from build123d import *

# Parameters (mm, degrees)
SKETCH2_R           = 42.538
SKETCH2_R_2         = 40.538
BOSS_EXTRUDE1_DEPTH = 51
CUT_EXTRUDE1_DEPTH  = 48
CUT_EXTRUDE3_START  = -1
CUT_EXTRUDE3_DEPTH  = 1
SKETCH29_R          = 10.65
CUT_EXTRUDE16_DEPTH = 1
CUT_EXTRUDE17_START = -2
SKETCH30_R          = 42.538
SKETCH30_R_2        = 41.538
CUT_EXTRUDE17_DEPTH = 2
BOSS_EXTRUDE3_DEPTH = 1
BOSS_EXTRUDE4_START = 1
SKETCH33_R          = 42.538
SKETCH33_R_2        = 41.638
BOSS_EXTRUDE4_DEPTH = 1


# Read off the part's stored shape, not the designer's step: Cut-Extrude3
with BuildPart() as part:
    # Sketch2 → Boss-Extrude1 (new body)
    with BuildSketch(Plane(origin=(0, 0, 0), x_dir=(-1, 0, 0), z_dir=(0, 1, 0))):
        with Locations(Location((-29.391570254, 2.611368154, 0), (0, 0, 90))):
            Circle(SKETCH2_R)
        with Locations(Location((-29.391570254, 2.611368154, 0), (0, 0, 90))):
            Circle(SKETCH2_R_2, mode=Mode.SUBTRACT)
    extrude(amount=BOSS_EXTRUDE1_DEPTH)

    # Sketch3 → Cut-Extrude1 (cut)
    with BuildSketch(Plane.XY):
        with BuildLine():
            Line((17.725570254, 19.5), (17.725570254, 51))
            Line((17.725570254, 51), (41.057570254, 51))
            Line((41.057570254, 51), (41.057570254, 19.5))
            ThreePointArc((41.057570254, 19.5), (29.391570254, 7.834), (17.725570254, 19.5))
        make_face()
    extrude(amount=CUT_EXTRUDE1_DEPTH, mode=Mode.SUBTRACT)

    # Cut-Extrude3 outline → Cut-Extrude3 (cut)
    with BuildSketch(Plane(origin=(0, 51, 0), x_dir=(1, 0, 0), z_dir=(0, 1, 0)).offset(CUT_EXTRUDE3_START)):
        with BuildLine():
            ThreePointArc((41.057570254, -43.518407744), (29.391570254, 39.926631846), (17.725570254, -43.518407744))
            Line((17.725570254, -43.518407744), (17.725570254, -41.434478385))
            ThreePointArc((17.725570254, -41.434478385), (29.391570254, 37.926631846), (41.057570254, -41.434478385))
            Line((41.057570254, -41.434478385), (41.057570254, -43.518407744))
        make_face()
    extrude(amount=CUT_EXTRUDE3_DEPTH, mode=Mode.SUBTRACT)

    # Sketch29 → Cut-Extrude16 (cut)
    with BuildSketch(Plane(origin=(58.783140508, 50, 5.222736308), x_dir=(1, 0, 0), z_dir=(0, 1, 0))):
        with Locations((-54.559325107, 32.628524909)):
            Circle(SKETCH29_R)
        with Locations((-4.223815401, 32.628524909)):
            Circle(SKETCH29_R)
        with Locations((5.046553517, -16.055747722)):
            Circle(SKETCH29_R)
        with Locations((-63.829694025, -16.055747722)):
            Circle(SKETCH29_R)
    extrude(amount=-CUT_EXTRUDE16_DEPTH, mode=Mode.SUBTRACT)

    # Sketch30 → Cut-Extrude17 (cut)
    with BuildSketch(Plane(origin=(0, 50, 0), x_dir=(1, 0, 0), z_dir=(0, 1, 0)).offset(CUT_EXTRUDE17_START)):
        with Locations(Location((29.391570254, -2.611368154, 0), (0, 0, 285.917258926))):
            Circle(SKETCH30_R)
        with Locations((29.391570254, -2.611368154)):
            Circle(SKETCH30_R_2, mode=Mode.SUBTRACT)
    extrude(amount=CUT_EXTRUDE17_DEPTH, mode=Mode.SUBTRACT)

    # Sketch32 → Boss-Extrude3 (add)
    with BuildSketch(Plane(origin=(0, 48, 0), x_dir=(1, 0, 0), z_dir=(0, 1, 0))):
        with BuildLine():
            Line((29.891570254, 38.923622444), (29.891570254, 39.923693196))
            ThreePointArc((29.891570254, 39.923693196), (29.391570254, 39.926631846), (28.891570254, 39.923693196))
            Line((28.891570254, 39.923693196), (28.891570254, 38.923622444))
            ThreePointArc((28.891570254, 38.923622444), (29.391570254, 38.926631846), (29.891570254, 38.923622444))
        make_face()
    extrude(amount=BOSS_EXTRUDE3_DEPTH)

    # Sketch33 → Boss-Extrude4 (add)
    with BuildSketch(Plane.XZ.offset(BOSS_EXTRUDE4_START)):
        with Locations(Location((29.391570254, 2.611368154, 0), (0, 0, 270))):
            Circle(SKETCH33_R)
        with Locations(Location((29.391570254, 2.611368154, 0), (0, 0, 270))):
            Circle(SKETCH33_R_2, mode=Mode.SUBTRACT)
    extrude(amount=-BOSS_EXTRUDE4_DEPTH)


solid = part.part
Could you check a few things on this model? Use its own coordinates, in mm. A direction names the side the tool comes from. Give positions to 0.01 mm unless a question says otherwise; leave off trailing zeros. Order: outer loops, then holes, each group sorted by start corner. A loop starts at its lowest first (then second) coordinate and runs counter-clockwise, first axis right, second up.
Item 1: If we section it at D-D, the plane y = 29: Write out the boundary of the cut face in (x, z), plus the area to 3 significant figures.
Item 2: For faces 1 (the face through (-11, 0, 12)), 2 (the face through (-12.6, 48, -1)), 3 (the face through (41.058, 35, 42)), 4 (the face through (31.053, 48.764, -38.893)), which set-ups out of +Z, -Z, +X, -X, +Y, -Y let a thin tool reach every point of the face, with its end or its side?
Item 3: If we section it at B-B, the plane z = -9: Write out the boundary of the cut face in (x, y).
Item 4: I need wall thicknesses on line 1 (Z direction, x = -6, y = 45.5); line 2 (X direction, y = 43.5, z = -28); line 3 (Z direction, x = 62.5, y = 4). Which ranges of each line are inside material? Lowest first, please.
Item 5: If we section it at A-A, the plane x = 53: Write out the boundary of the cut face in (y, z).
Item 6: If we section it at C-C, the plane x = 21: Write out the boundary of the cut face in (y, z) (3 decimals), plus the area to 3 significant figures.
Item 7: I'm going to push flat-ended pins straight in: pin 1 (16 mm diameter, centred on x = 4.5, z = -29, fed in from +Y); pin 2 (12 mm diameter, centred on x = 48.5, y = 5, fed in from +Z); pin 3 (2.5 mm diameter, centred on y = 39.5, z = 42, fed in from -X); pin 4 (12 mm diameter, centred on x = 16.5, z = -26.5, fed in from +Y). Where does each tip first touch, or does it pass through?
Values:
1. outline: (17.73, 41.43) - (17.73, 43.52) arc R42.54 ccw (long way) to (41.06, 43.52) - (41.06, 41.43) arc R40.54 cw (long way) to start
1. area: 475 mm2
2. face 1: -Y
2. face 2: -X, +Y
2. face 3: +Z, +Y
2. face 4: +Y
3. outline: (-11.53, -1) - (-10.59, -1) - (-10.59, 0) - (-9.45, 0) - (-9.45, 50) - (-10.49, 50) - (-10.49, 48) - (-11.53, 48) - close; (68.23, 0) - (69.38, 0) - (69.38, -1) - (70.31, -1) - (70.31, 48) - (69.27, 48) - (69.27, 50) - (68.23, 50) - close
4. line 1: z = -20.99 to -17.16, 22.38 to 26.21
4. line 2: x = -0.15 to 2.82, 55.97 to 58.93
4. line 3: z = -24.1 to -20.78, 26 to 29.32
5. outline: (-1, -32.77) - (48, -32.77) - (48, -31.57) - (49, -31.57) - (49, -30.34) - (0, -30.34) - (0, -31.69) - (-1, -31.69) - close; (-1, 36.91) - (0, 36.91) - (0, 35.57) - (50, 35.57) - (50, 36.79) - (48, 36.79) - (48, 38) - (-1, 38) - close
6. outline: (-1, -39.091) - (48, -39.091) - (48, -38.07) - (50, -38.07) - (50, -37.049) - (0, -37.049) - (0, -38.172) - (-1, -38.172) - close; (-1, 43.395) - (0, 43.395) - (0, 42.271) - (11.396, 42.271) - (11.396, 44.313) - (-1, 44.313) - close
6. area: 125 mm2
7. pin 1: stops at y = 49
7. pin 2: stops at z = 43.08
7. pin 3: stops at x = 10.55
7. pin 4: passes through
